Geometry check sheet. Reference: the model listing, model coordinates, mm. A direction names the side the tool comes from. Coordinates: 2 decimals unless noted, no trailing zeros. Loops run counter-clockwise (first coordinate to the right, second up) from the corner with the lowest first, then second, coordinate; pieces in that order, holes last. Notation, with made-up numbers: (76, -12) -> (81, -12) arc R29 cw to (81, 22) -> close; hole circle Ø10 at (-34, 17). An arc over 180 degrees is marked (long way). Answer as a JSON object with one key per item and string values.
from build123d import *

# Parameters (mm, degrees)
SKETCH1_W                      = 13
SKETCH1_H                      = 8
BOSS_EXTRUDE1_DEPTH            = 3.8
SKETCH2_R                      = 0.95
BOSS_EXTRUDE2_DEPTH            = 5.6
BOSS_EXTRUDE5_DEPTH            = 3.8
CBORE_FOR_M3_SHCS1_D           = 3.4
CBORE_FOR_M3_SHCS1_CBORE_D     = 6.5
CBORE_FOR_M3_SHCS1_CBORE_DEPTH = 3.2
CHAMFER4_SIZE                  = 0.4


with BuildPart() as part:
    # Sketch1 → Boss-Extrude1 (new body)
    with BuildSketch(Plane(origin=(0, 0, 0), x_dir=(1, 0, 0), z_dir=(0, 1, 0))):
        Rectangle(SKETCH1_W, SKETCH1_H)
    extrude(amount=BOSS_EXTRUDE1_DEPTH)

    # Sketch2 → Boss-Extrude2 (add)
    with BuildSketch(Plane.XZ):
        with Locations((3.25, 1)):
            Circle(SKETCH2_R)
        with Locations((-3.25, 1)):
            Circle(SKETCH2_R)
    extrude(amount=BOSS_EXTRUDE2_DEPTH)

    # Sketch8 → Boss-Extrude5 (add)
    with BuildSketch(Plane(origin=(0, 3.8, 0), x_dir=(1, 0, 0), z_dir=(0, 1, 0))):
        Polygon((-9.5, -13.63), (9.5, -13.63), (9.5, -8.815), (13.5, -8.815), (13.5, -0.815), (9.5, -0.815), (9.5, 4), (-9.5, 4), align=None)
    extrude(amount=-BOSS_EXTRUDE5_DEPTH)

    # CBORE for M3 SHCS1 (through all)
    with Locations(Plane(origin=(0, 3.8, 0), x_dir=(1, 0, 0), z_dir=(0, 1, 0))):
        with Locations((9.5, -4.815)):
            CounterBoreHole(CBORE_FOR_M3_SHCS1_D / 2, CBORE_FOR_M3_SHCS1_CBORE_D / 2, CBORE_FOR_M3_SHCS1_CBORE_DEPTH)

    # Chamfer4
    chamfer4_edges = [part.edges().sort_by_distance(p)[0] for p in [
        (2.3, -5.6, 1),
        (-4.2, -5.6, 1),
        (-9.5, 3.8, 4.815),
        (0, 3.8, 13.63),
        (9.5, 3.8, 11.2225),
        (11.5, 3.8, 8.815),
        (13.5, 3.8, 4.815),
        (11.5, 3.8, 0.815),
        (9.5, 3.8, -1.5925),
        (-9.5, 1.9, -4),
        (-9.5, 0, 4.815),
        (-9.5, 1.9, 13.63),
        (0, 0, 13.63),
        (9.5, 1.9, 13.63),
        (9.5, 0, 11.2225),
        (9.5, 1.9, 8.815),
        (11.5, 0, 8.815),
        (13.5, 1.9, 8.815),
        (13.5, 0, 4.815),
        (13.5, 1.9, 0.815),
        (11.5, 0, 0.815),
        (9.5, 1.9, 0.815),
        (9.5, 0, -1.5925),
        (9.5, 1.9, -4),
        (0, 0, -4),
        (0, 3.8, -4),
    ]]
    chamfer(chamfer4_edges, length=CHAMFER4_SIZE)


solid = part.part
1. Section check C-C, the plane y = -0.75. Record the boundary of the cut face in (x, z), then the cut area to 3 significant figures.
Evaluation:
{"outline": "circle Ø1.9 at (-3.25, 1); circle Ø1.9 at (3.25, 1)", "area": "5.67 mm^2"}
2. Section check D-D, the plane x = 5.5. Record the boundary of the cut face in (y, z), then the cut area to 3 significant figures.
Evaluation:
{"outline": "(0, -3.6) -> (0.4, -4) -> (3.4, -4) -> (3.8, -3.6) -> (3.8, 13.23) -> (3.4, 13.63) -> (0.4, 13.63) -> (0, 13.23) -> close", "area": "66.7 mm^2"}
3. Section check B-B, the plane z = 12.75. Record the boundary of the cut face in (x, y), then the cut area to 3 significant figures.
Evaluation:
{"outline": "(-9.5, 0.4) -> (-9.1, 0) -> (9.1, 0) -> (9.5, 0.4) -> (9.5, 3.4) -> (9.1, 3.8) -> (-9.1, 3.8) -> (-9.5, 3.4) -> close", "area": "71.9 mm^2"}
4. Depth check by flat-ended pin: P1, Ø0.9, axis at y = 2, z = -1, coming from the +X side; P2, Ø5, axis at x = 6, y = -3, coming from the -Z side; P3, Ø1.5, axis at x = 11, y = 2, coming from the -Z side (3 decimals). Enter the tip coordinate at first touch or a pass-through.
Evaluation:
{"P1": "stops at x = 9.5", "P2": "stops at z = 0.08", "P3": "stops at z = 0.815"}
5. Mould release check, pull along X, two halves, no side actions. Record for faces 5 (the face through (6.253, 2.222, 4.672)), 6 (the face through (-9.5, 2, 5)), 7 (the face through (12, 2, 0.815)): released by +X, released by -X, zero draft, split by the parting line, or undercut.
Evaluation:
{"face 5": "undercut", "face 6": "released by -X", "face 7": "zero draft"}
6. Tool access check on faces 1 (the face through (11, 0.6, 6)), 2 (the face through (2.3, -2.6, 1)), 3 (the face through (9.5, 2, -2)), 4 (the face through (9.5, 2, 11)). Record the directions out of +Z, -Z, +X, -X, +Y, -Y that give a thin tool (end or side, any length) a straight path to the whole face; none if there is none.
Evaluation:
{"face 1": "+Y", "face 2": "-Y", "face 3": "-Z, +X, +Y, -Y", "face 4": "+Z, +X, +Y, -Y"}
7. Section check A-A, the plane x = -3.25. Record the boundary of the cut face in (y, z), then the cut area to 3 significant figures.
Evaluation:
{"outline": "(-5.6, 0.45) -> (-5.2, 0.05) -> (0, 0.05) -> (0, -3.6) -> (0.4, -4) -> (3.4, -4) -> (3.8, -3.6) -> (3.8, 13.23) -> (3.4, 13.63) -> (0.4, 13.63) -> (0, 13.23) -> (0, 1.95) -> (-5.2, 1.95) -> (-5.6, 1.55) -> close", "area": "77.2 mm^2"}
8. Thickness scan on probe 1 along X at (y, z) = (2, 0.25); probe 2 along Y at (x, z) = (0.5, -1); probe 3 along Z at (x, y) = (9.5, 0.35) (3 decimals). Record the ranges inside material, lowest first. Write a range as from..to.
Evaluation:
{"probe 1": "x = -9.5..9.5", "probe 2": "y = 0..3.8", "probe 3": "z = 0.465..3.115, 6.515..9.165"}
